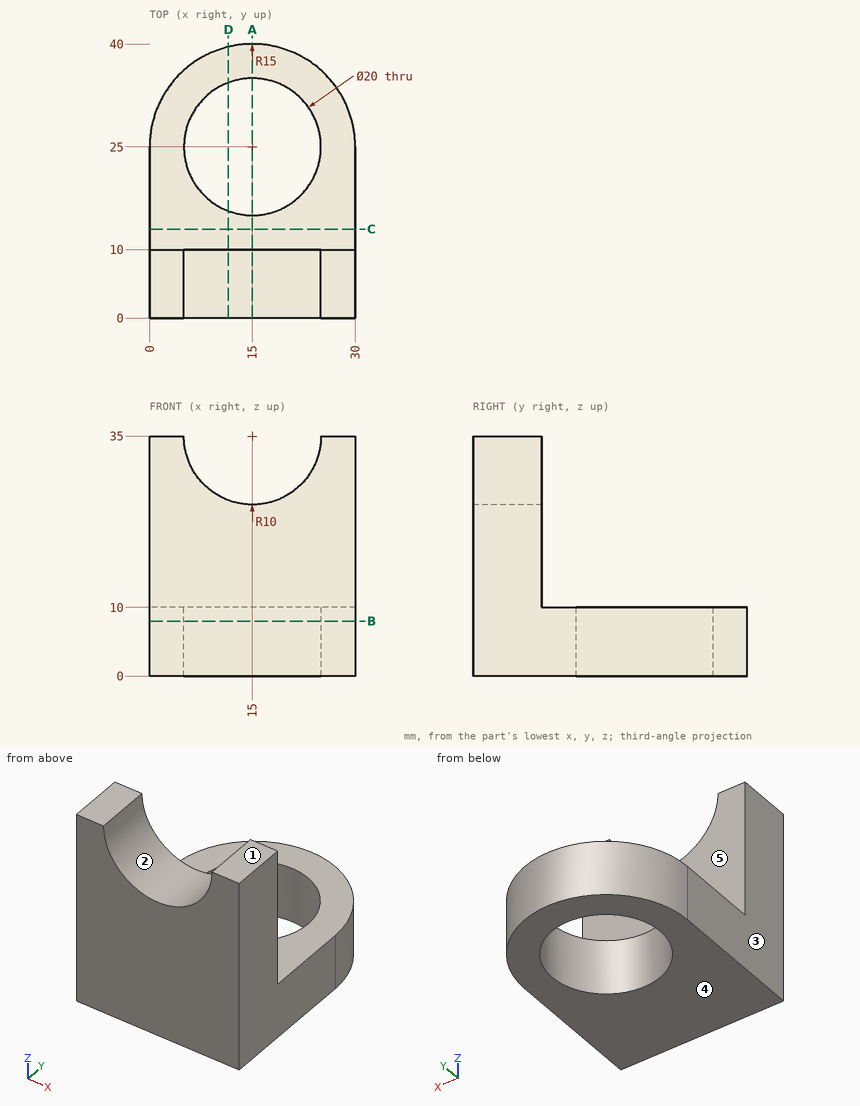
Verification items for this drawing (mm, ordinates from the low corner). A direction names the side the tool comes from. Round coordinates to 2 decimals unless told otherwise and drop trailing zeros. Loops run counter-clockwise (first coordinate to the right, second up) from the corner with the lowest first, then second, coordinate; pieces in that order, holes last. Notation, with made-up numbers: M -27,39.25 L 27,39.25 A29 cw 27,72.25 Z; hole C 39.25,-37 d8. An arc over 180 degrees is marked long. Answer as a JSON object with one key per item and string values.
1. Gauge pin test, flat ends, axial feed: P1, Ø15, axis at x = 13.5, y = 31, coming from the +Z side; P2, Ø6, axis at x = 17, y = 19, coming from the +Z side; P3, Ø4, axis at y = 31, z = 11, coming from the +X side; P4, Ø5, axis at x = 21, z = 25.5, coming from the -Y side. Record the tip position at first contact, or that the pin passes through.
Reply:
{"P1": "stops at z = 10", "P2": "passes through", "P3": "stops at x = 29.38", "P4": "stops at y = 0"}
2. Mould release check, pull along X, two halves, no side actions. Record for the marked faces 1, 2 and 3: pulls with the +X half, pulls with the -X half, needs draft (parallel to the pull), parting line crosses it, or undercut.
Reply:
{"face 1": "needs draft", "face 2": "undercut", "face 3": "pulls with the -X half"}
3. Section check A-A (x = 15). Record the boundary of the cut face in (y, z).
Reply:
{"outline": "M 0,0 L 15,0 L 15,10 L 10,10 L 10,25 L 0,25 Z; M 35,0 L 40,0 L 40,10 L 35,10 Z"}
4. Section check D-D (x = 11.5). Record the boundary of the cut face in (y, z), plus the area to 3 significant figures.
Reply:
{"outline": "M 0,0 L 15.63,0 L 15.63,10 L 10,10 L 10,25.63 L 0,25.63 Z; M 34.37,0 L 39.59,0 L 39.59,10 L 34.37,10 Z", "area": "365 mm²"}
5. Scan lines: line 1 (Y direction, x = 15, z = 5); line 2 (Z direction, x = 21.25, y = 34). Record each from-to range of solid material in increasing order.
Reply:
{"line 1": "y = 0 to 15, 35 to 40", "line 2": "z = 0 to 10"}
6. Section check C-C (y = 13). Record the boundary of the cut face in (x, z), plus the area to 3 significant figures.
Reply:
{"outline": "M 0,0 L 30,0 L 30,10 L 0,10 Z", "area": "300 mm²"}
7. Access from +Z, -Z, +X, -X, +Y, -Y to the whole of each face (thin tool, end or side, straight path). Record for the marked faces 4 and 5.
Reply:
{"face 4": "-Z, +X, -X, +Y, -Y", "face 5": "+Z, +X, -X, +Y"}
8. Section check B-B (z = 8). Record the boundary of the cut face in (x, y).
Reply:
{"outline": "M 0,0 L 30,0 L 30,25 A15 ccw 0,25 Z; hole C 15,25 d20"}
